The model under review builds one solid part; all positions refer to its coordinate system, in mm. A direction names the side the tool comes from. Give positions to 0.01 mm unless a question says otherwise; leave off trailing zeros. Order: outer loops, then holes, each group sorted by start corner. A loop starts at its lowest first (then second) coordinate and runs counter-clockwise, first axis right, second up. Notation, with made-up numbers: (40, -31) - (88, -31) arc R10 cw to (88, -21) - close; hole circle Ø7 at (12, 30.5). An arc over 180 degrees is marked (long way). Write item = value, one per line. Start each with the question number.
1. We need section A-A, the plane z = 484. Give the boundary of the cut face in (x, y) (3 decimals), and give its area (3 significant figures).
2. For P1, Ø10.5, axis at x = -28.575, z = 914.4, coming from the +Y side; P2, Ø10.5, axis at x = -16.5, z = 413.5, coming from the -Y side (3 decimals); P3, Ø5, axis at y = -30.5, z = 320.5, coming from the -X side (3 decimals), all flat-tipped, find the tip position at first contact; note any pin that passes through.
3. Machinability: for faces 1 (the flat face through (-21, -3.175, 501)), 2 (the flat face through (-11, -2, 1016)), which of the approach directions +Z, -Z, +X, -X, +Y, -Y give a long, thin tool a straight path to every point of the face, cutting with its end or side? Answer none if there is none.
4. We need section B-B, the plane x = -16. Give the boundary of the cut face in (y, z) (3 decimals), and give its area (3 significant figures).
5. Wall thickness on probe 1 along X at (y, z) = (-1, 711); probe 2 along Y at (x, z) = (-27, 937) (3 decimals): over which ranges is each line inside the solid? List them lowest first.
from build123d import *

# Parameters (mm, degrees)
BOSS_EXTRUDE1_DEPTH = 1016
SKETCH4_R           = 3.96875
CUT_EXTRUDE3_DEPTH  = 44.45
LPATTERN1_COUNT     = 5
LPATTERN1_PITCH     = 203.2


with BuildPart() as part:
    # Sketch1 → Boss-Extrude1 (new body)
    with BuildSketch(Plane.XY):
        Polygon((0, 0), (-38.1, 0), (-38.1, -3.175), (-3.175, -3.175), (-3.175, -38.1), (0, -38.1), align=None)
    extrude(amount=BOSS_EXTRUDE1_DEPTH)

    # Sketch4 → Cut-Extrude3 (cut)
    with BuildSketch(Plane(origin=(10.670100368, 3.175, 791.563272881), x_dir=(1, 0, 0), z_dir=(0, 1, 0))):
        with Locations((-39.245100368, 689.963272881)):
            Circle(SKETCH4_R)
    cut_extrude3 = extrude(amount=-CUT_EXTRUDE3_DEPTH, mode=Mode.SUBTRACT)

    # LPattern1: Cut-Extrude3 ×5, 1 skipped
    with Locations(*[(0, 0, i * LPATTERN1_PITCH) for i in range(1, LPATTERN1_COUNT) if i not in (2,)]):
        add(cut_extrude3, mode=Mode.SUBTRACT)


solid = part.part
Model answer:
q1.outline = (-38.1, -3.175) - (-3.175, -3.175) - (-3.175, -38.1) - (0, -38.1) - (0, 0) - (-38.1, 0) - close
q1.area = 232 mm2
q2.P1 = 0
q2.P2 = -3.175
q2.P3 = -3.175
q3.face_1 = +Z, -Z, -X, -Y
q3.face_2 = +Z, +X, -X, +Y, -Y
q4.outline = (-3.175, 0) - (0, 0) - (0, 1016) - (-3.175, 1016) - close
q4.area = 3,230 mm2
q5.probe_1 = -38.1 to -32.54, -24.61 to 0
q5.probe_2 = -3.175 to 0
